```python
from build123d import *

# Parameters (mm, degrees)
POCKET060_DEPTH       = 100
SKETCH263_R           = 2
PAD089_DEPTH          = 4
POLARPATTERN001_COUNT = 4


with BuildPart() as part:
    # Sketch113 → Revolution002 (revolve)
    with BuildSketch(Plane.XZ):
        with BuildLine():
            ThreePointArc((0, 16), (-22.1147575162, 14.8720734917), (-44, 11.5))
            Line((-44, 11.5), (-44, 16))
            Line((-44, 16), (-60, 16))
            Line((-60, 16), (-60, 18))
            Line((0, 18), (-60, 18))
            Line((0, 16), (0, 18))
        make_face()
    revolve(axis=Axis((0, 0, 0), (0, 0, 1)))

    # Sketch114 → Pocket060 (cut)
    with BuildSketch(Plane.XY):
        with BuildLine():
            Line((-12, 16), (12, 16))
            ThreePointArc((16, 12), (14.8284271247, 14.8284271247), (12, 16))
            Line((16, 12), (16, -12))
            ThreePointArc((12, -16), (14.8284271247, -14.8284271247), (16, -12))
            Line((12, -16), (-12, -16))
            ThreePointArc((-16, -12), (-14.8284271247, -14.8284271247), (-12, -16))
            Line((-16, -12), (-16, 12))
            ThreePointArc((-12, 16), (-14.8284271247, 14.8284271247), (-16, 12))
        make_face()
    extrude(amount=POCKET060_DEPTH, mode=Mode.SUBTRACT)

    # Sketch263 → Pad089 (join)
    with BuildSketch(Plane.XY.offset(14.5)):
        with Locations((25.4558441227, 25.4558441227)):
            Circle(SKETCH263_R)
    pad089 = extrude(amount=-PAD089_DEPTH)

    # PolarPattern001: Pad089 ×4 about axis
    polarpattern001_axis = Axis((0, 0, 14.5), (0, 0, 1))
    for i in range(1, POLARPATTERN001_COUNT):
        add(pad089.rotate(polarpattern001_axis, i * 360 / POLARPATTERN001_COUNT))


solid = part.part
```
The model under review builds one solid part; all positions refer to its coordinate system, in mm. A direction names the side the tool comes from. Give positions to 0.01 mm unless a question says otherwise; leave off trailing zeros. Write each loop counter-clockwise with the first axis right and the second up, starting at its lowest first coordinate (ties: lowest second). Pieces come first, ordered by that corner, then holes. Notation, with made-up numbers: M -27,-15 L 31,-15 A7 ccw 31,-6 Z; hole C 3,58.5 d5. An arc over 180 degrees is marked long. Write item = value, one per line. Start each with the question number.
Q1. For line 1 (Z direction, x = 25, y = -51.5); line 2 (X direction, y = -8, z = 17.5); line 3 (Z direction, x = -32, y = -30), list the stretches that pass through material, from the lowest coordinate up.
Q2. We need section C-C (x = 36). State the section outline as (y, z) points.
Q3. Mouldability with a two-part tool opening along X and no side actions: class faces 1 (the face through (-25, -25, 10.5)), 2 (the face through (0, 16, 17)), 3 (the face through (59.94, -2.64, 17.01)) as released by +X, released by -X, zero draft, split by the parting line, or undercut.
Q4. Machinability: for faces 4 (the face through (9.538, 42.954, 13.782)), 5 (the face through (-14.797, 14.859, 16.472)), 6 (the face through (25, -25, 10.5)), which of the approach directions +Z, -Z, +X, -X, +Y, -Y give a long, thin tool a straight path to every point of the face, cutting with its end or side? Answer none if there is none.
Q5. Clearance check with flat-ended pins moving along their axes: pin 1 (3 mm diameter, centred on y = 37, z = 14, fed in from +X); pin 2 (4 mm diameter, centred on x = -13, y = -24.5, fed in from -Z); pin 3 (1.5 mm diameter, centred on y = -3, z = 17, fed in from +X). State where each tip first meets the part, or that it passes through.
Q6. We need section A-A (x = 0). State the section outline as (y, z) points, plus the area to 3 significant figures.
Result set:
q1.line_1 = 16 to 18
q1.line_2 = -59.46 to -16, 16 to 59.46
q1.line_3 = 11.53 to 18
q2.outline = M -48,16 L -25.3,16 L -25.3,11.5 A214.36 cw 25.3,11.5 L 25.3,16 L 48,16 L 48,18 L -48,18 Z
q3.face_1 = zero draft
q3.face_2 = undercut
q3.face_3 = split by the parting line
q4.face_4 = -Z
q4.face_5 = +Z, -Z
q4.face_6 = -Z, +X, -X, +Y, -Y
q5.pin_1 = 26
q5.pin_2 = 13.96
q5.pin_3 = 59.96
q6.outline = M -60,16 L -44,16 L -44,11.5 A217.36 cw -16,15.41 L -16,18 L -60,18 Z; M 16,15.41 A217.36 cw 44,11.5 L 44,16 L 60,16 L 60,18 L 16,18 Z
q6.area = 301 mm2
